Autodesk Inventor part; units mm, degrees
ref_plane "YZ Plane" through (0, 0, 0) normal (1, 0, 0) x (0, 1, 0)
ref_plane "XZ Plane" through (0, 0, 0) normal (0, 1, 0) x (-1, 0, 0)
ref_plane "XY Plane" through (0, 0, 0) normal (0, 0, 1) x (1, 0, 0)
sketch "Sketch1" plane through (0, 0, 0) normal (0, 0, 1) x (1, 0, 0)
  line L0 (0, 0) -> (220, 0)
  line L1 (220, 0) -> (220, 220)
  line L2 (220, 220) -> (0, 220)
  line L3 (0, 220) -> (0, 0)
  line L4 (5.5, 214.5) -> (214.5, 214.5) construction
  line L5 (214.5, 214.5) -> (214.5, 5.5) construction
  line L6 (214.5, 5.5) -> (5.5, 5.5) construction
  line L7 (5.5, 5.5) -> (5.5, 214.5) construction
  circle A0 centre (5.5, 5.5) radius 1.6
  circle A1 centre (5.5, 214.5) radius 1.6
  circle A2 centre (214.5, 214.5) radius 1.6
  circle A3 centre (214.5, 5.5) radius 1.6
  line L8 (165, 87.2183) -> (132.7817, 55)
  line L9 (132.7817, 55) -> (87.2183, 55)
  line L10 (87.2183, 55) -> (55, 87.2183)
  line L11 (55, 87.2183) -> (55, 132.7817)
  line L12 (55, 132.7817) -> (87.2183, 165)
  line L13 (132.7817, 165) -> (165, 132.7817)
  line L14 (165, 132.7817) -> (165, 87.2183)
  line L15 (150, 126.5685) -> (150, 93.4315)
  line L16 (150, 93.4315) -> (126.5685, 70)
  line L17 (126.5685, 70) -> (93.4315, 70)
  line L18 (93.4315, 70) -> (70, 93.4315)
  line L19 (70, 93.4315) -> (70, 126.5685)
  line L20 (70, 126.5685) -> (93.4315, 150)
  line L21 (93.4315, 150) -> (126.5685, 150)
  line L22 (126.5685, 150) -> (150, 126.5685)
  line L23 (205, 205) -> (205, 15)
  line L24 (205, 15) -> (15, 15)
  line L25 (15, 15) -> (15, 205)
  line L26 (102.5, 165) -> (102.5, 205)
  line L27 (117.5, 205) -> (117.5, 165)
  line L28 (15, 205) -> (102.5, 205)
  line L29 (117.5, 205) -> (205, 205)
  line L30 (87.2183, 165) -> (102.5, 165)
  line L31 (117.5, 165) -> (132.7817, 165)
  point P0 (214.5, 110)
  point P1 (220, 110)
  point P2 (110, 214.5)
  point P3 (110, 220)
  point P4 (110, 110)
  point P5 (110, 110)
  dimension "d0" = 220
  dimension "d1" = 220
  dimension "d2" = 209
  dimension "d3" = 209
  dimension "d4" = 3.2
  dimension "d5" = 3.2
  dimension "d6" = 3.2
  dimension "d7" = 3.2
  dimension "d9" = 15
  dimension "d10" = 15
  dimension "d11" = 15
  dimension "d12" = 15
  dimension "d13" = 15
  dimension "d14" = 80
  dimension "d15" = 7.5
extrude "Extrusion1" add sketch "Sketch1" along normal blind 6.5
sketch "Sketch2" plane through (0, 0, 6.5) normal (0, 0, 1) x (1, 0, 0)
  line L0 (205, 205) -> (205, 15)
  line L1 (205, 15) -> (15, 15)
  line L2 (15, 15) -> (15, 205)
  line L3 (55, 87.2183) -> (87.2183, 55)
  line L4 (132.7817, 55) -> (165, 87.2183)
  line L5 (0, 220) -> (0, 0)
  line L6 (65.8058, 76.4124) -> (15, 25.6066)
  line L7 (76.4124, 65.8058) -> (25.6066, 15)
  line L8 (143.5876, 65.8058) -> (194.3934, 15)
  line L9 (154.1942, 76.4124) -> (205, 25.6066)
  line L10 (205, 25.6066) -> (205, 15)
  line L11 (205, 15) -> (194.3934, 15)
  line L12 (15, 25.6066) -> (15, 15)
  line L13 (15, 15) -> (25.6066, 15)
  line L14 (15, 15) -> (71.1091, 71.1091) construction
  line L15 (148.8909, 71.1091) -> (205, 15) construction
  line L16 (65.8058, 76.4124) -> (76.4124, 65.8058)
  line L17 (143.5876, 65.8058) -> (154.1942, 76.4124)
  dimension "d18" = 15
  dimension "d19" = 15
  dimension "d20" = 7.5
  dimension "d21" = 7.5
extrude "Extrusion2" add sketch "Sketch2" against normal blind 6.5
sketch "Sketch4" plane through (0, 0, 6.5) normal (0, 0, 1) x (1, 0, 0)
  line L0 (93.4315, 150) -> (126.5685, 150)
  line L1 (0, 0) -> (220, 0)
  line L2 (220, 0) -> (220, 220)
  line L3 (220, 220) -> (0, 220)
  line L4 (0, 220) -> (0, 0)
  line L5 (-23.9453, -6) -> (243.9453, -6) construction
  line L6 (-23.9453, -6) -> (110, 226) construction
  line L7 (110, 226) -> (243.9453, -6) construction
  circle A0 centre (110, 226) radius 2.75
  circle A1 centre (243.9453, -6) radius 2.75
  circle A2 centre (-23.9453, -6) radius 2.75
  arc A3 (-30.4405, -2.25) -> (-22.5946, -13.3774) centre (-23.9453, -6) ccw
  arc A4 (116.4952, 229.75) -> (103.5048, 229.75) centre (110, 226) ccw
  arc A5 (242.5946, -13.3774) -> (250.4405, -2.25) centre (243.9453, -6) ccw
  line L8 (122.1244, 220) -> (116.4952, 229.75)
  line L9 (103.5048, 229.75) -> (97.8756, 220)
  line L10 (0, 50.4744) -> (-30.4405, -2.25)
  line L11 (250.4405, -2.25) -> (220, 50.4744)
  line L12 (242.5946, -13.3774) -> (169.5256, 0)
  line L13 (-22.5946, -13.3774) -> (50.4744, 0)
  line L14 (0, 50.4744) -> (0, 0)
  line L15 (0, 0) -> (50.4744, 0)
  line L16 (169.5256, 0) -> (220, 0)
  line L17 (220, 50.4744) -> (220, 0)
  point P0 (110, 150)
  dimension "d30" = 5.5
  dimension "d31" = 5.5
  dimension "d32" = 5.5
  dimension "d33" = 15
  dimension "d34" = 15
  dimension "d35" = 15
  dimension "d36" = 6
  dimension "d37" = 6
extrude "Extrusion3" add sketch "Sketch4" against normal blind 6.5 contours L1 L13 A3 L10 L4 | L1 L2 L11 A5 L12 | L9 A4 L8 L3
chamfer "Chamfer1" distance 4 angle 45 16 edges at (25.6066, 15, 3.25) (15, 25.6066, 3.25) (76.4124, 65.8058, 3.25) (65.8058, 76.4124, 3.25) (194.3934, 15, 3.25) (205, 25.6066, 3.25) (143.5876, 65.8058, 3.25) (154.1942, 76.4124, 3.25) (117.5, 205, 3.25) (102.5, 205, 3.25) (117.5, 165, 3.25) (102.5, 165, 3.25) (205, 205, 3.25) (15, 205, 3.25) (0, 220, 3.25) (220, 220, 3.25)
sketch "Sketch5" plane through (0, 0, 6.5) normal (0, 0, 1) x (1, 0, 0)
  line L0 (117.5, 169) -> (117.5, 201)
  line L1 (28.435, 17.8284) -> (29.6066, 15)
  line L2 (15, 29.6066) -> (17.8284, 28.435)
  line L3 (102.5, 201) -> (102.5, 169)
  line L4 (93.4315, 150) -> (126.5685, 150)
  line L5 (0, 216) -> (4, 220)
  line L6 (220, 50.4744) -> (220, 216)
  line L7 (70, 126.5685) -> (150, 93.4315) construction
  line L8 (150, 126.5685) -> (70, 93.4315) construction
  line L9 (102.5, 150) -> (102.5, 106)
  line L10 (102.5, 106) -> (106, 102.5)
  line L11 (106, 102.5) -> (114, 102.5)
  line L12 (114, 102.5) -> (117.5, 106)
  line L13 (117.5, 106) -> (117.5, 150)
  circle A0 centre (110, 110) radius 1.5
  point P0 (0, 0)
  dimension "d43" = 3
  dimension "d44" = 8
  dimension "d45" = 7.5
  dimension "d46" = 7.5
extrude "Extrusion4" add sketch "Sketch5" against normal blind 6.5
chamfer "Chamfer2" distance 4 angle 45 2 edges at (102.5, 150, 3.25) (117.5, 150, 3.25)
equation "\"d5\" = d4"
equation "\"d6\" = d4"
equation "\"d7\" = d4"
equation "\"d31\" = d30"
equation "\"d32\" = d30"
equation "\"d34\" = d33"
equation "\"d35\" = d33"
equation "\"d46\" = d45"
properties part number "heatbed_mount_v3"
Check sheet for the modelled part. Datum: model origin and axes. Units: mm. A direction names the side the tool comes from. Round coordinates to 2 decimals unless told otherwise and drop trailing zeros. Write each loop counter-clockwise with the first axis right and the second up, starting at its lowest first coordinate (ties: lowest second). Pieces come first, ordered by that corner, then holes. Notation, with made-up numbers: (54, 62) -> (101, 62) arc R15 ccw to (101, 86) -> close; hole circle Ø11 at (-19, 38.25). An arc over 180 degrees is marked (long way). Answer as CSV lines item,"result". Start each with the question number.
1) Go/stop test with flat-tipped pins: P1, Ø3, axis at y = 117, z = 4.5, coming from the +X side; P2, Ø2, axis at x = 16, z = 3.5, coming from the -Y side; P3, Ø3, axis at x = 182, z = 3, coming from the -Y side. Record where each tip stops, or that it passes through.
2) Section check A-A on x = 39.5. Enter the section's corners in (y, z), and give its area (3 significant figures).
3) Tool access check on faces 1 (the flat face through (62.977, 76, 3)), 2 (the cylindrical face through (110.1, 233.5, 3.3)), 3 (the flat face through (170, 220, 3)). Record the directions out of +Z, -Z, +X, -X, +Y, -Y that give a thin tool (end or side, any length) a straight path to the whole face; none if there is none.
4) Section check C-C on z = 5. State how many separate pieces and enclosed holes the cut face has, and give its area (3 significant figures).
5) Section check B-B on y = 178.5. Enter the section's corners in (x, z), and give its area (4 significant figures).
6) Release check for a two-part mould opening along X. For faces 4 (the flat face through (52, 220, 3)), 5 (the flat face through (0, 134, 3)), 6 (the flat face through (110, 55, 3)), 7 (the flat face through (220, 132, 3)) record: pulls with the +X half, pulls with the -X half, needs draft (parallel to the pull), parting line crosses it, or undercut.
7) Material ranges on line 1 (X direction, y = 214.5, z = 2); line 2 (X direction, y = 183.5, z = 5); line 3 (Y direction, x = 46.5, z = 1), recorded low to high. Write a range as from..to.
Found:
1,P1,"stops at x = 220"
1,P2,"stops at y = -6.49"
1,P3,"stops at y = -2.56"
2,outline,"(-2.01, 0) -> (15, 0) -> (15, 6.5) -> (-2.01, 6.5) -> close; (28.89, 0) -> (50.11, 0) -> (50.11, 6.5) -> (28.89, 6.5) -> close; (205, 0) -> (220, 0) -> (220, 6.5) -> (205, 6.5) -> close"
2,area,"346 mm^2"
3,face 1,"+Z, -Z"
3,face 2,"+Z, -Z, +Y"
3,face 3,"+Z, -Z, +X, +Y"
4,separate pieces,"1"
4,enclosed holes,"12"
4,area,"23,500 mm^2"
5,outline,"(0, 0) -> (15, 0) -> (15, 6.5) -> (0, 6.5) -> close; (102.5, 0) -> (117.5, 0) -> (117.5, 6.5) -> (102.5, 6.5) -> close; (205, 0) -> (220, 0) -> (220, 6.5) -> (205, 6.5) -> close"
5,area,"292.5 mm^2"
6,face 4,"needs draft"
6,face 5,"pulls with the -X half"
6,face 6,"undercut"
6,face 7,"pulls with the +X half"
7,line 1,"x = 0..3.9, 7.1..212.9, 216.1..220"
7,line 2,"x = 0..15, 102.5..117.5, 205..220"
7,line 3,"y = -0.73..15, 35.89..57.11, 205..220"
